from build123d import *

# Parameters (mm, degrees)
SKETCH1_W                      = 100
SKETCH1_H                      = 100
SKETCH1_W_2                    = 94
SKETCH1_H_2                    = 94
EXTRUDE_THIN1_DEPTH            = 130
FILLET1_R                      = 0.5
FILLET2_R                      = 3
F_8_0_8_DIAMETER_HOLE2_D       = 8
F_8_0_8_DIAMETER_HOLE3_D       = 8
F_10_0_10_DIAMETER_HOLE1_D     = 10
F_10_0_10_DIAMETER_HOLE2_D     = 10
F_6_0_6_DIAMETER_HOLE1_D       = 6
F_6_0_6_DIAMETER_HOLE1_DEPTH   = 3
F_6_0_6_DIAMETER_HOLE2_D       = 6
F_6_0_6_DIAMETER_HOLE2_DEPTH   = 3
F_21_0_21_DIAMETER_HOLE1_D     = 21
F_21_0_21_DIAMETER_HOLE1_DEPTH = 3
F_5_0_5_DIAMETER_HOLE1_D       = 5
F_5_0_5_DIAMETER_HOLE1_DEPTH   = 3
F_8_0_8_DIAMETER_HOLE4_D       = 8
F_8_0_8_DIAMETER_HOLE4_DEPTH   = 3
CUT_EXTRUDE1_REACH             = 173.464
SKETCH31_R                     = 2
SKETCH31_R_2                   = 3.5
F_8_0_8_DIAMETER_HOLE5_D       = 8
F_8_0_8_DIAMETER_HOLE5_DEPTH   = 3


with BuildPart() as part:
    # Sketch1 → Extrude-Thin1 (new body)
    with BuildSketch(Plane.XY):
        Rectangle(SKETCH1_W, SKETCH1_H)
        Rectangle(SKETCH1_W_2, SKETCH1_H_2, mode=Mode.SUBTRACT)
    extrude(amount=EXTRUDE_THIN1_DEPTH)

    # Fillet1
    fillet1_edges = [part.edges().sort_by_distance(p)[0] for p in [
        (47, -47, 65),
        (47, 47, 65),
        (-47, 47, 65),
        (-47, -47, 65),
    ]]
    fillet(fillet1_edges, radius=FILLET1_R)

    # Fillet2
    fillet2_edges = [part.edges().sort_by_distance(p)[0] for p in [
        (50, -50, 65),
        (-50, -50, 65),
        (-50, 50, 65),
        (50, 50, 65),
    ]]
    fillet(fillet2_edges, radius=FILLET2_R)

    # Ø8.0 (8) Diameter Hole2 (through all)
    with Locations(Plane(origin=(0, 50, 0), x_dir=(1, 0, 0), z_dir=(0, 1, 0))):
        with Locations((28, -32), (28, -90)):
            Hole(F_8_0_8_DIAMETER_HOLE2_D / 2)

    # Ø8.0 (8) Diameter Hole3 (through all)
    with Locations(Plane(origin=(50, 0, 0), x_dir=(0, 0, -1), z_dir=(1, 0, 0))):
        with Locations((-14, 31), (-110, 31)):
            Hole(F_8_0_8_DIAMETER_HOLE3_D / 2)

    # Ø10.0 (10) Diameter Hole1 (through all)
    with Locations(Plane(origin=(0, 50, 0), x_dir=(1, 0, 0), z_dir=(0, 1, 0))):
        with Locations((-34, -56)):
            Hole(F_10_0_10_DIAMETER_HOLE1_D / 2)

    # Ø10.0 (10) Diameter Hole2 (through all)
    with Locations(Plane(origin=(50, 0, 0), x_dir=(0, 0, -1), z_dir=(1, 0, 0))):
        with Locations((-44, -31)):
            Hole(F_10_0_10_DIAMETER_HOLE2_D / 2)

    # Ø6.0 (6) Diameter Hole1
    with Locations(Plane.ZY.offset(50)):
        with Locations((56, -15), (56, 35)):
            Hole(F_6_0_6_DIAMETER_HOLE1_D / 2, depth=F_6_0_6_DIAMETER_HOLE1_DEPTH)

    # Ø6.0 (6) Diameter Hole2
    with Locations(Plane(origin=(0, -50, 0), x_dir=(-1, 0, 0), z_dir=(0, -1, 0))):
        with Locations((20, -44), (-35, -44)):
            Hole(F_6_0_6_DIAMETER_HOLE2_D / 2, depth=F_6_0_6_DIAMETER_HOLE2_DEPTH)

    # Ø21.0 (21) Diameter Hole1
    with Locations(Plane(origin=(50, 0, 0), x_dir=(0, 0, -1), z_dir=(1, 0, 0))):
        with Locations((-70, 0)):
            Hole(F_21_0_21_DIAMETER_HOLE1_D / 2, depth=F_21_0_21_DIAMETER_HOLE1_DEPTH)

    # Ø5.0 (5) Diameter Hole1
    with Locations(Plane(origin=(50, 0, 0), x_dir=(0, 0, -1), z_dir=(1, 0, 0))):
        with Locations((-41.157258279, -16.652364697), (-53.347635303, 28.842741721), (-98.842741721, 16.652364697), (-86.652364697, -28.842741721)):
            Hole(F_5_0_5_DIAMETER_HOLE1_D / 2, depth=F_5_0_5_DIAMETER_HOLE1_DEPTH)

    # Ø8.0 (8) Diameter Hole4
    with Locations(Plane(origin=(0, 50, 0), x_dir=(1, 0, 0), z_dir=(0, 1, 0))):
        with Locations((-3, -25)):
            Hole(F_8_0_8_DIAMETER_HOLE4_D / 2, depth=F_8_0_8_DIAMETER_HOLE4_DEPTH)

    # Sketch31 → Cut-Extrude1 (cut, up to next)
    with BuildSketch(Plane(origin=(50, 0, 0), x_dir=(0, 0, -1), z_dir=(1, 0, 0)), mode=Mode.PRIVATE) as cut_extrude1_sk1:
        with Locations(Location((-5, 4, 0), (0, 0, 90))):
            Circle(SKETCH31_R)
    cut_extrude1_tool1 = extrude(cut_extrude1_sk1.sketch, amount=-CUT_EXTRUDE1_REACH, mode=Mode.PRIVATE) & part.part
    # Sketch31 → Cut-Extrude1 (cut, up to next)
    with BuildSketch(Plane(origin=(50, 0, 0), x_dir=(0, 0, -1), z_dir=(1, 0, 0)), mode=Mode.PRIVATE) as cut_extrude1_sk2:
        with Locations(Location((-5, 13, 0), (0, 0, 90))):
            Circle(SKETCH31_R)
    cut_extrude1_tool2 = extrude(cut_extrude1_sk2.sketch, amount=-CUT_EXTRUDE1_REACH, mode=Mode.PRIVATE) & part.part
    # Sketch31 → Cut-Extrude1 (cut, up to next)
    with BuildSketch(Plane(origin=(50, 0, 0), x_dir=(0, 0, -1), z_dir=(1, 0, 0)), mode=Mode.PRIVATE) as cut_extrude1_sk3:
        with Locations(Location((-125, 13, 0), (0, 0, 90))):
            Circle(SKETCH31_R)
    cut_extrude1_tool3 = extrude(cut_extrude1_sk3.sketch, amount=-CUT_EXTRUDE1_REACH, mode=Mode.PRIVATE) & part.part
    # Sketch31 → Cut-Extrude1 (cut, up to next)
    with BuildSketch(Plane(origin=(50, 0, 0), x_dir=(0, 0, -1), z_dir=(1, 0, 0)), mode=Mode.PRIVATE) as cut_extrude1_sk4:
        with Locations(Location((-125, 4, 0), (0, 0, 90))):
            Circle(SKETCH31_R)
    cut_extrude1_tool4 = extrude(cut_extrude1_sk4.sketch, amount=-CUT_EXTRUDE1_REACH, mode=Mode.PRIVATE) & part.part
    # Sketch31 → Cut-Extrude1 (cut, up to next)
    with BuildSketch(Plane(origin=(50, 0, 0), x_dir=(0, 0, -1), z_dir=(1, 0, 0)), mode=Mode.PRIVATE) as cut_extrude1_sk5:
        with Locations(Location((-23, 8.5, 0), (0, 0, 90))):
            Circle(SKETCH31_R_2)
    cut_extrude1_tool5 = extrude(cut_extrude1_sk5.sketch, amount=-CUT_EXTRUDE1_REACH, mode=Mode.PRIVATE) & part.part
    # Sketch31 → Cut-Extrude1 (cut, up to next)
    with BuildSketch(Plane(origin=(50, 0, 0), x_dir=(0, 0, -1), z_dir=(1, 0, 0)), mode=Mode.PRIVATE) as cut_extrude1_sk6:
        with Locations(Location((-107, 8.5, 0), (0, 0, 90))):
            Circle(SKETCH31_R_2)
    cut_extrude1_tool6 = extrude(cut_extrude1_sk6.sketch, amount=-CUT_EXTRUDE1_REACH, mode=Mode.PRIVATE) & part.part
    add(cut_extrude1_tool1.solids().sort_by_distance((50, 4, 5))[0], mode=Mode.SUBTRACT)
    add(cut_extrude1_tool2.solids().sort_by_distance((50, 13, 5))[0], mode=Mode.SUBTRACT)
    add(cut_extrude1_tool3.solids().sort_by_distance((50, 13, 125))[0], mode=Mode.SUBTRACT)
    add(cut_extrude1_tool4.solids().sort_by_distance((50, 4, 125))[0], mode=Mode.SUBTRACT)
    add(cut_extrude1_tool5.solids().sort_by_distance((50, 8.5, 23))[0], mode=Mode.SUBTRACT)
    add(cut_extrude1_tool6.solids().sort_by_distance((50, 8.5, 107))[0], mode=Mode.SUBTRACT)

    # Ø8.0 (8) Diameter Hole5
    with Locations(Plane(origin=(0, 50, 0), x_dir=(1, 0, 0), z_dir=(0, 1, 0))):
        with Locations((-33, -25)):
            Hole(F_8_0_8_DIAMETER_HOLE5_D / 2, depth=F_8_0_8_DIAMETER_HOLE5_DEPTH)


solid = part.part
Input: part model. Units: mm. Frame: model coordinates. A direction names the side the tool comes from. Round coordinates to 2 decimals unless told otherwise and drop trailing zeros. Order: outer loops, then holes, each group sorted by start corner. A loop starts at its lowest first (then second) coordinate and runs counter-clockwise, first axis right, second up.
1. Pin query (flat end, axial travel): P1, Ø5, axis at y = 35, z = 56, coming from the -X side; P2, Ø5, axis at y = 31, z = 14, coming from the -X side; P3, Ø3.5, axis at y = 4, z = 125, coming from the +X side; P4, Ø1, axis at x = 34, z = 44.5, coming from the -Y side. Return the tip coordinate at first contact, or that it passes through.
The answers:
P1: stops at x = 47
P2: passes through
P3: stops at x = -47
P4: stops at y = 47
2. Cut plane B-B, the plane y = 40. Output: boundary loops of the cut face in (x, z), then the cut area to 3 significant figures.
The answers:
outline: (-50, 0) - (-47, 0) - (-47, 130) - (-50, 130) - close; (47, 0) - (50, 0) - (50, 130) - (47, 130) - close
area: 780 mm2
3. Cut plane D-D, the plane y = -33. Output: boundary loops of the cut face in (x, z), then the cut area to 3 significant figures.
The answers:
outline: (-50, 0) - (-47, 0) - (-47, 39.42) - (-50, 39.42) - close; (-50, 48.58) - (-47, 48.58) - (-47, 130) - (-50, 130) - close; (47, 0) - (50, 0) - (50, 39.42) - (47, 39.42) - close; (47, 48.58) - (50, 48.58) - (50, 130) - (47, 130) - close
area: 725 mm2
4. Set-up query: faces 1 (the face through (32.79, -48.48, 41.97)), 2 (the face through (-48, -15, 59)), 3 (the face through (48.521, 5.92, 25.365)). Return all of +Z, -Z, +X, -X, +Y, -Y with unobstructed straight access to the full face (end or side cutting, diameter ignored); none if empty.
The answers:
face 1: -Y
face 2: -X
face 3: +X
5. Mould query, pull axis Y, two halves, no side actions, for faces 4 (the face through (-30, -49, 53)), 5 (the face through (-1, 50, 64)), 6 (the face through (49.1, -49.14, 65.91)), 7 (the face through (48.479, 34.966, 109.479)). Classes: released by +Y, released by -Y, zero draft, split by the parting line, or undercut.
The answers:
face 4: zero draft
face 5: released by +Y
face 6: released by -Y
face 7: undercut
6. Cut plane A-A, the plane z = 5. Output: boundary loops of the cut face in (x, y).
The answers:
outline: (-50, -47) arc R3 ccw to (-47, -50) - (47, -50) arc R3 ccw to (50, -47) - (50, 2) - (47, 2) - (47, -46.5) arc R0.5 cw to (46.5, -47) - (-46.5, -47) arc R0.5 cw to (-47, -46.5) - (-47, 46.5) arc R0.5 cw to (-46.5, 47) - (46.5, 47) arc R0.5 cw to (47, 46.5) - (47, 15) - (50, 15) - (50, 47) arc R3 ccw to (47, 50) - (-47, 50) arc R3 ccw to (-50, 47) - close; (47, 6) - (50, 6) - (50, 11) - (47, 11) - close
7. Material intervals for line 1 (Y direction, x = -34.5, z = 70.5); line 2 (Z direction, x = 28, y = -48.5), sorted ascending.
The answers:
line 1: y = -50 to -47, 47 to 50
line 2: z = 0 to 28, 36 to 86, 94 to 130
